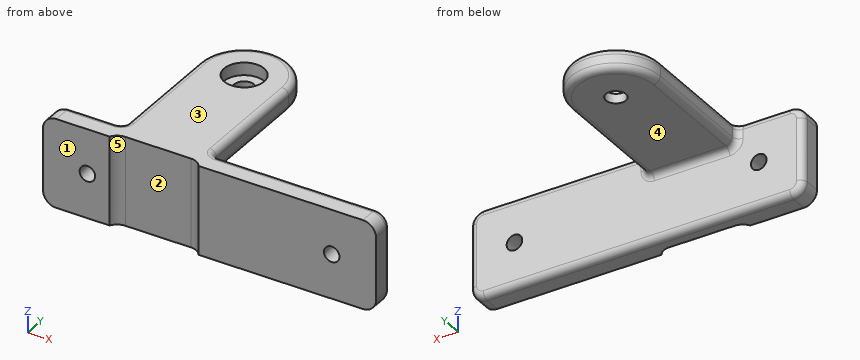
```python
from build123d import *

# Parameters (mm, degrees)
SKETCH1_W                               = 150
SKETCH1_H                               = 40
BASE_PLATE_DEPTH                        = 10
VERT_BOSS_DEPTH                         = 10
SKETCH5_W                               = 40
SKETCH5_H                               = 3
SLOT_DEPTH                              = 177.988700204
F_7_0_7_DIAMETER_HOLE1_D                = 7
CBORE_FOR_M8_HEX_HEAD_BOLT1_D           = 9
CBORE_FOR_M8_HEX_HEAD_BOLT1_CBORE_D     = 18.01
CBORE_FOR_M8_HEX_HEAD_BOLT1_CBORE_DEPTH = 5.68
FILLET1_R                               = 6
FILLET2_R                               = 3


with BuildPart() as part:
    # Sketch1 → Base Plate (new body)
    with BuildSketch(Plane(origin=(0, 0, 0), x_dir=(1, 0, 0), z_dir=(0, 1, 0))):
        with Locations((75, 20)):
            Rectangle(SKETCH1_W, SKETCH1_H)
    extrude(amount=BASE_PLATE_DEPTH)

    # Sketch2 → Vert Boss (add)
    with BuildSketch(Plane.XY):
        with BuildLine():
            Line((30, 0), (30, 65))
            ThreePointArc((30, 65), (50, 85), (70, 65))
            Line((70, 65), (70, 0))
            Line((70, 0), (30, 0))
        make_face()
    extrude(amount=-VERT_BOSS_DEPTH)

    # Sketch5 → Slot (cut, through all)
    with BuildSketch(Plane.XY):
        with Locations((50, 1.5)):
            Rectangle(SKETCH5_W, SKETCH5_H)
    extrude(amount=-SLOT_DEPTH, mode=Mode.SUBTRACT)

    # Ø7.0 (7) Diameter Hole1 (through all)
    with Locations(Plane(origin=(0, 10, 0), x_dir=(-1, 0, 0), z_dir=(0, 1, 0))):
        with Locations((-130, -20), (-20, -20)):
            Hole(F_7_0_7_DIAMETER_HOLE1_D / 2)

    # CBORE for M8 Hex Head Bolt1 (through all)
    with Locations(Plane.XY):
        with Locations((50, 65)):
            CounterBoreHole(CBORE_FOR_M8_HEX_HEAD_BOLT1_D / 2, CBORE_FOR_M8_HEX_HEAD_BOLT1_CBORE_D / 2, CBORE_FOR_M8_HEX_HEAD_BOLT1_CBORE_DEPTH)

    # Fillet1
    # the kernel refuses this fillet: 6 mm, written as the material it adds along each edge
    with BuildSketch(Plane(origin=(70, 3, 0), x_dir=(-1, 0, 0), z_dir=(0, 0, -1))) as fillet1_piece_1:
        with BuildLine():
            CenterArc((5.196152423, -6), FILLET1_R, 90, 60)
            Line((0, -3), (0, 0))
            Line((0, 0), (5.196152423, 0))
        make_face()
    extrude(amount=40)
    with BuildSketch(Plane(origin=(30, 3, 0), x_dir=(0, -1, 0), z_dir=(0, 0, -1))) as fillet1_piece_2:
        with BuildLine():
            CenterArc((6, -5.196152423), FILLET1_R, 120, 60)
            Line((0, -5.196152423), (0, 0))
            Line((0, 0), (3, 0))
        make_face()
    extrude(amount=40)
    # the kernel refuses this fillet: 6 mm, written as the material it takes off along each edge
    with BuildSketch(Plane(origin=(0, -15, 0), x_dir=(1, 0, 0), z_dir=(0, 1, 0)), Plane(origin=(0, -15, -40), x_dir=(0, 0, 1), z_dir=(0, 1, 0))) as fillet1_2_piece_1:
        with BuildLine():
            CenterArc((FILLET1_R, FILLET1_R), FILLET1_R, 180, 90)
            Line((0, FILLET1_R), (0, 0))
            Line((0, 0), (FILLET1_R, 0))
        make_face()
    extrude(amount=40, mode=Mode.SUBTRACT)
    with BuildSketch(Plane(origin=(150, -15, -40), x_dir=(0, 0, 1), z_dir=(0, 1, 0)), Plane(origin=(150, -15, 0), x_dir=(-1, 0, 0), z_dir=(0, 1, 0))) as fillet1_2_piece_2:
        with BuildLine():
            CenterArc((FILLET1_R, -FILLET1_R), FILLET1_R, 90, 90)
            Line((0, -FILLET1_R), (0, 0))
            Line((0, 0), (FILLET1_R, 0))
        make_face()
    extrude(amount=40, mode=Mode.SUBTRACT)

    # Fillet2
    fillet2_edges = [part.edges().sort_by_distance(p)[0] for p in [
        (107, 10, 0),
        (30, 37.5, -10),
        (70, 37.5, -10),
        (30, 37.5, 0),
        (70, 37.5, 0),
        (50, 85, 0),
        (30, 10, -5),
        (50, 85, -10),
        (70, 10, -5),
        (50, 10, -10),
        (18, 10, 0),
        (0, 10, -20),
        (150, 10, -20),
        (75, 10, -40),
        (148.242640687, 10, -1.757359313),
        (148.242640687, 10, -38.242640687),
        (1.757359313, 10, -38.242640687),
        (1.757359313, 10, -1.757359313),
    ]]
    fillet(fillet2_edges, radius=FILLET2_R)


solid = part.part
```
The listing builds one solid part. Answer for the finished solid, in the listing's coordinates (mm). Face numbers are marked on the shaded views. A direction names the side the tool comes from. Coordinates: 2 decimals unless noted, no trailing zeros. Loops run counter-clockwise (first coordinate to the right, second up) from the corner with the lowest first, then second, coordinate; pieces in that order, holes last. Notation, with made-up numbers: (27, 71.25) - (69, 71.25) arc R24 cw to (69, 94.25) - close; hole circle Ø10 at (19.5, 2.5). An arc over 180 degrees is marked (long way). Write item = value, one per line.
1) Determine the mould class of the marked faces 1 and 2 for opening direction X: pulls with the +X half, pulls with the -X half, needs draft (parallel to the pull), parting line crosses it, or undercut.
Responses:
face_1 = needs draft
face_2 = undercut
2) Which of the six approach directions +Z, -Z, +X, -X, +Y, -Y give full straight-line access (tool end or side, diameter ignored) to the marked faces 3, 4 and 5?
Responses:
face_3 = +Z, +X, -X, +Y, -Y
face_4 = -Z, +X, -X, +Y
face_5 = +Z, -Z, -Y
3) Section D-D (z = -28.5) is taken. Determine the outline of the cut face in (x, y), plus the area to 3 significant figures.
Responses:
outline = (0, 0) - (30, 0) arc R6 cw to (35.2, 3) - (64.8, 3) arc R6 cw to (70, 0) - (150, 0) - (150, 7) arc R3 ccw to (147, 10) - (3, 10) arc R3 ccw to (0, 7) - close
area = 1,390 mm^2
4) Section B-B (z = -20) is taken. Determine the outline of the cut face in (x, y).
Responses:
outline = (0, 0) - (16.5, 0) - (16.5, 10) - (3, 10) arc R3 ccw to (0, 7) - close; (23.5, 0) - (30, 0) arc R6 cw to (35.2, 3) - (64.8, 3) arc R6 cw to (70, 0) - (126.5, 0) - (126.5, 10) - (23.5, 10) - close; (133.5, 0) - (150, 0) - (150, 7) arc R3 ccw to (147, 10) - (133.5, 10) - close
5) Section C-C (y = 26.5) is taken. Determine the outline of the cut face in (x, z), plus the area to 3 significant figures.
Responses:
outline = (30, -7) arc R3 ccw to (33, -10) - (67, -10) arc R3 ccw to (70, -7) - (70, -3) arc R3 ccw to (67, 0) - (33, 0) arc R3 ccw to (30, -3) - close
area = 392 mm^2
6) Find the intervals of material crossed by line 1 along Z through (x, y) = (130, 4); line 2 along Y through (x, z) = (37.5, -27); line 3 along Y through (x, z) = (104, -23), in increasing order.
Responses:
line_1 = -40 to -23.5, -16.5 to 0
line_2 = 3 to 10
line_3 = 0 to 10
7) Section A-A (x = 50) is taken. Determine the outline of the cut face in (y, z) (3 decimals).
Responses:
outline = (3, -40) - (7, -40) arc R3 ccw to (10, -37) - (10, -13) arc R3 cw to (13, -10) - (60.5, -10) - (60.5, -5.68) - (55.995, -5.68) - (55.995, 0) - (3, 0) - close; (69.5, -10) - (82, -10) arc R3 ccw to (85, -7) - (85, -3) arc R3 ccw to (82, 0) - (74.005, 0) - (74.005, -5.68) - (69.5, -5.68) - close
8) Each of these flat-tipped pins is pushed along its axis until it touches: P1, Ø5.5, axis at x = 53.5, y = 62.5, coming from the +Z side; P2, Ø3, axis at y = 43.5, z = -5.5, coming from the +X side; P3, Ø5.5, axis at x = 20, z = -20, coming from the +Y side; P4, Ø4, axis at x = 83, y = 10, coming from the -Z side. Where does it stop, or does it pass through?
Responses:
P1 = -5.68
P2 = 70
P3 = through
P4 = -39.83
